```python
from build123d import *

# Parameters (mm, degrees)
SKETCH1_W                = 92
SKETCH1_H                = 68
BOSS_EXTRUDE1_DEPTH      = 18
SKETCH2_R                = 8
CUT_EXTRUDE4_DEPTH       = 18
BOSS_EXTRUDE3_DEPTH      = 92
FILLET2_R                = 6
BOSS_EXTRUDE4_DEPTH      = 37
BOSS_EXTRUDE4_DEPTH_BACK = 18
SKETCH9_R                = 40
SKETCH10_R               = 20
CUT_EXTRUDE6_DEPTH       = 90
RIB6_START               = -7
RIB6_DEPTH               = 14
FILLET3_R                = 6


# Read off the part's stored shape, not the designer's step: Rib6
with BuildPart() as part:
    # Sketch1 → Boss-Extrude1 (new body)
    with BuildSketch(Plane.XY):
        Rectangle(SKETCH1_W, SKETCH1_H)
    extrude(amount=BOSS_EXTRUDE1_DEPTH)

    # Sketch2 → Cut-Extrude4 (cut)
    with BuildSketch(Plane(origin=(0, 0, 0), x_dir=(-1, 0, 0), z_dir=(0, 0, -1))):
        with Locations((-18, -14)):
            Circle(SKETCH2_R)
        with Locations(Location((18, -14, 0), (0, 0, 180))):
            Circle(SKETCH2_R)
    extrude(amount=-CUT_EXTRUDE4_DEPTH, mode=Mode.SUBTRACT)

    # Sketch7 → Boss-Extrude3 (add)
    with BuildSketch(Plane.ZY.offset(46)):
        with BuildLine():
            Line((0, 28), (-35, 28))
            ThreePointArc((-35, 28), (-47.727922061, 33.272077939), (-53, 46))
            Line((-53, 46), (-53, 93))
            Line((-53, 93), (-65, 93))
            Line((-65, 93), (-65, 34))
            ThreePointArc((-65, 34), (-59.727922061, 21.272077939), (-47, 16))
            Line((-47, 16), (-6, 16))
            ThreePointArc((-6, 16), (-1.757359313, 17.757359313), (0, 22))
            Line((0, 22), (0, 28))
        make_face()
    extrude(amount=-BOSS_EXTRUDE3_DEPTH)

    # Fillet2
    fillet2_edges = [part.edges().sort_by_distance(p)[0] for p in [
        (0, 28, 0),
    ]]
    fillet(fillet2_edges, radius=FILLET2_R - 0.0001)  # a hair under: the kernel refuses the full size

    # Sketch9 → Boss-Extrude4 (add, two sides: drawn at the far end of the back side and taken through both)
    with BuildSketch(Plane(origin=(0, 0, -65), x_dir=(-1, 0, 0), z_dir=(0, 0, -1)).offset(-BOSS_EXTRUDE4_DEPTH_BACK)):
        with Locations((0, 93)):
            Circle(SKETCH9_R)
    extrude(amount=BOSS_EXTRUDE4_DEPTH + BOSS_EXTRUDE4_DEPTH_BACK)

    # Sketch10 → Cut-Extrude6 (cut)
    with BuildSketch(Plane(origin=(0, 0, -102), x_dir=(-1, 0, 0), z_dir=(0, 0, -1))):
        with Locations((0, 93)):
            Circle(SKETCH10_R)
    extrude(amount=-CUT_EXTRUDE6_DEPTH, mode=Mode.SUBTRACT)

    # Rib6 outline → Rib6 (add)
    with BuildSketch(Plane(origin=(0, 0, 0), x_dir=(0, 0, -1), z_dir=(1, 0, 0)).offset(RIB6_START)):
        with BuildLine():
            Line((89, 54), (65, 54))
            Line((65, 54), (65, 34))
            ThreePointArc((65, 34), (59.727922061, 21.272077939), (47, 16))
            Line((47, 16), (6, 16))
            ThreePointArc((6, 16), (1.757359313, 17.757359313), (0, 22))
            Line((0, 22), (0, -34))
            Line((0, -34), (66.284356879, 0.259330522))
            ThreePointArc((66.284356879, 0.259330522), (82.874384935, 15.729386584), (89, 37.570368832))
            Line((89, 37.570368832), (89, 54))
        make_face()
    extrude(amount=RIB6_DEPTH)

    # Fillet3
    fillet3_edges = [part.edges().sort_by_distance(p)[0] for p in [
        (0, 53, -89),
    ]]
    fillet(fillet3_edges, radius=FILLET3_R)


solid = part.part
```
The listing builds one solid part. Answer for the finished solid, in the listing's coordinates (mm). A direction names the side the tool comes from. Give positions to 0.01 mm unless a question says otherwise; leave off trailing zeros. Order: outer loops, then holes, each group sorted by start corner. A loop starts at its lowest first (then second) coordinate and runs counter-clockwise, first axis right, second up. Notation, with made-up numbers: (-10, -7.75) -> (32, -7.75) arc R20 ccw to (32, 1.25) -> close; hole circle Ø3 at (-24, 2.5). An arc over 180 degrees is marked (long way). Answer as a JSON object with one key per item and string values. Group by question number.
Item 1: Flat-ended cylindrical pins translate along their axes: pin 1 (20 mm diameter, centred on x = -13, z = 5.5, fed in from +Y); pin 2 (8 mm diameter, centred on x = 0, y = 43, fed in from -Z); pin 3 (4 mm diameter, centred on x = -16, z = -48.5, fed in from -Y). Find the tip coordinate at first contact, or state that the pin passes through.
Item 2: Determine the mould class of faces 1 (the cylindrical face through (0.644, 29.804, -1.711)), 2 (the flat face through (-1, -34, 9)), 3 (the cylindrical face through (-0.644, 33.133, -47.587)) for opening direction Y: pulls with the +Y half, pulls with the -Y half, needs draft (parallel to the pull), parting line crosses it, or undercut.
Item 3: The part is cut by section C-C on z = -77. Write down the section's boundary in (x, y), and give its area (3 significant figures).
Item 4: The part is cut by section B-B on y = -14. Write down the section's boundary in (x, z).
Item 5: Consider L1, parallel to Y at x = -18, z = 14; L2, parallel to Z at x = 8, y = 67.5; L3, parallel to X at y = 102, z = -87. Determine where each line is inside the solid, lowest interval first. Write a range as from..to.
Item 6: The part is cut by section A-A on x = 18. Give the number of separate pieces and of enclosed holes in the cut face, and give its area (3 significant figures).
Item 7: A tool of negligible diameter and unlimited length cuts with its end or side. For faces 4 (the flat face through (-1, 28, -20)), 5 (the cylindrical face through (26.227, 21.413, -59.867)), 6 (the flat face through (9.4, 111.3, -47)), 7 (the flat face through (-43, 93, -59)), 8 (the flat face through (-31, 51, -65)), from which of +Z, -Z, +X, -X, +Y, -Y can it reach the whole face along a straight path? Write none if from no direction.
Result set:
{
 "1": {"pin 1": "y = 34", "pin 2": "z = -89", "pin 3": "y = 16"},
 "2": {"face 1": "pulls with the +Y half", "face 2": "pulls with the -Y half", "face 3": "undercut"},
 "3": {"outline": "(-7, 8.18) -> (7, 8.18) -> (7, 53.62) arc R40 ccw (long way) to (-7, 53.62) -> close; hole circle Ø40 at (0, 93)", "area": "4,400 mm²"},
 "4": {"outline": "(-46, 0) -> (-26, 0) -> (-26, 18) -> (-46, 18) -> close; (-10, 0) -> (-7, 0) -> (-7, -38.7) -> (7, -38.7) -> (7, 0) -> (10, 0) -> (10, 18) -> (-10, 18) -> close; (26, 0) -> (46, 0) -> (46, 18) -> (26, 18) -> close"},
 "5": {"L1": "-34..-22, -6..34", "L2": "-102..-47", "L3": "-38.97..-17.86, 17.86..38.97"},
 "6": {"separate pieces": "3", "enclosed holes": "0", "area": "5,040 mm²"},
 "7": {"face 4": "+X, -X, +Y", "face 5": "-Z, +X, -Y", "face 6": "+Z, +X, -X, +Y", "face 7": "+Z, -Z, -X, +Y", "face 8": "-Z, -X, -Y"}
}
